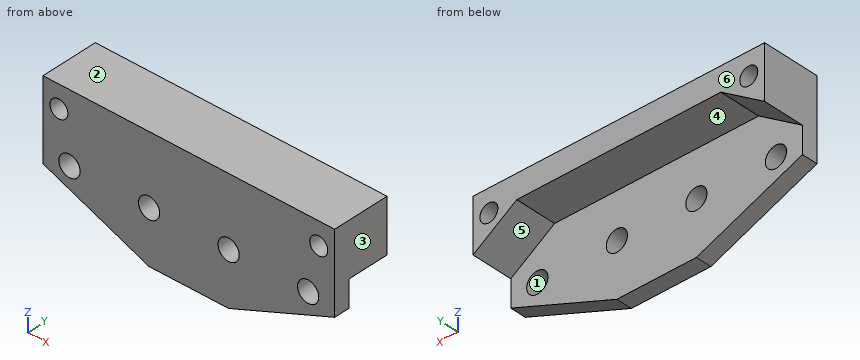
```python
from build123d import *

# Parameters (mm, degrees)
SKETCH2_R           = 2
BOSS_EXTRUDE1_DEPTH = 3
BOSS_EXTRUDE2_DEPTH = 7.8
SKETCH4_R           = 1.7
CUT_EXTRUDE1_DEPTH  = 61.585806919


with BuildPart() as part:
    # Sketch2 → Boss-Extrude1 (new body)
    with BuildSketch(Plane(origin=(0, 0, 0), x_dir=(1, 0, 0), z_dir=(0, 1, 0))):
        Polygon((0, 0), (0, 15), (20, 23), (35, 23), (55, 15), (55, 0), align=None)
        with Locations(Location((5, 13, 0), (0, 0, 270))):
            Circle(SKETCH2_R, mode=Mode.SUBTRACT)
        with Locations(Location((20, 13, 0), (0, 0, 270))):
            Circle(SKETCH2_R, mode=Mode.SUBTRACT)
        with Locations(Location((35, 13, 0), (0, 0, 270))):
            Circle(SKETCH2_R, mode=Mode.SUBTRACT)
        with Locations(Location((50, 13, 0), (0, 0, 270))):
            Circle(SKETCH2_R, mode=Mode.SUBTRACT)
    extrude(amount=BOSS_EXTRUDE1_DEPTH)

    # Sketch3 → Boss-Extrude2 (add)
    with BuildSketch(Plane(origin=(0, 3, 0), x_dir=(1, 0, 0), z_dir=(0, 1, 0))):
        Polygon((0, 10), (0, 0), (15, 0), (8.25, 4.5), align=None)
        Polygon((8.25, 4.5), (15, 0), (40, 0), (46.75, 4.5), align=None)
        Polygon((46.75, 4.5), (40, 0), (55, 0), (55, 10), align=None)
    extrude(amount=BOSS_EXTRUDE2_DEPTH)

    # Sketch4 → Cut-Extrude1 (cut, through all)
    with BuildSketch(Plane(origin=(0, 10.8, 0), x_dir=(1, 0, 0), z_dir=(0, 1, 0))):
        with Locations(Location((3, 4.25, 0), (0, 0, 270))):
            Circle(SKETCH4_R)
        with Locations(Location((52, 4.25, 0), (0, 0, 270))):
            Circle(SKETCH4_R)
    extrude(amount=-CUT_EXTRUDE1_DEPTH, mode=Mode.SUBTRACT)


solid = part.part
```
The model under review builds one solid part; all positions refer to its coordinate system, in mm. Face numbers are marked on the shaded views. A direction names the side the tool comes from. Coordinates: 2 decimals unless noted, no trailing zeros. Order: outer loops, then holes, each group sorted by start corner. A loop starts at its lowest first (then second) coordinate and runs counter-clockwise, first axis right, second up. Notation, with made-up numbers: (-10, 80) -> (20, 80) arc R23 ccw to (20, 100) -> close; hole circle Ø11 at (14.5, 68.5). An arc over 180 degrees is marked (long way). Answer in a Markdown table with one row per item. Add a question column.
Item 1: Machinability: for the marked faces 5 and 6, which of the approach directions +Z, -Z, +X, -X, +Y, -Y give a long, thin tool a straight path to every point of the face, cutting with its end or side? Answer none if there is none.
Item 2: We need section B-B on y = 8.75. Write out the cut boundary in (x, z).
Item 3: Mouldability with a two-part tool opening along Z and no side actions: class the marked faces 1, 2, 3 and 4 as +Z half, -Z half, draft (parallel to the pull), parting line (faces both ways), or undercut.
Item 4: We need section A-A on y = 1.25. Write out the cut boundary in (x, z), plus the area to 3 significant figures.
Item 5: Clearance check with flat-ended pins moving along their axes: pin 1 (4.5 mm diameter, centred on x = 5, z = -13, fed in from +Y); pin 2 (3 mm diameter, centred on x = 40, y = 8.5, fed in from -Z). State where each tip first meets the part, or that it passes through.
Item 6: We need section D-D on z = -11.5. Write out the cut boundary in (x, y).
Item 7: We need section C-C on x = 9.5. Write out the cut boundary in (y, z), plus the area to 3 significant figures.
Item 8: To check wall thickness, follow probe 1 along X at (y, z) = (2.3, -13); probe 2 along X at (y, z) = (5.25, -4.25); probe 3 along Y at (x, z) = (32, -21). State the ranges of each line that lie inside material, in increasing order.
Final values:
| question | item | result |
|---|---|---|
| 1 | face 5 | -Z, +Y |
| 1 | face 6 | +Z, -Z, +X, -X, +Y |
| 2 | outline | (0, -10) -> (8.25, -4.5) -> (46.75, -4.5) -> (55, -10) -> (55, 0) -> (0, 0) -> close; hole circle Ø3.4 at (3, -4.25); hole circle Ø3.4 at (52, -4.25) |
| 3 | face 1 | undercut |
| 3 | face 2 | +Z half |
| 3 | face 3 | draft |
| 3 | face 4 | -Z half |
| 4 | outline | (0, -15) -> (20, -23) -> (35, -23) -> (55, -15) -> (55, 0) -> (0, 0) -> close; hole circle Ø3.4 at (3, -4.25); hole circle Ø4 at (5, -13); hole circle Ø4 at (20, -13); hole circle Ø4 at (35, -13); hole circle Ø4 at (50, -13); hole circle Ø3.4 at (52, -4.25) |
| 4 | area | 1,040 mm2 |
| 5 | pin 1 | stops at y = 3 |
| 5 | pin 2 | stops at z = -4.5 |
| 6 | outline | (0, 0) -> (3.68, 0) -> (3.68, 3) -> (0, 3) -> close; (6.32, 0) -> (18.68, 0) -> (18.68, 3) -> (6.32, 3) -> close; (21.32, 0) -> (33.68, 0) -> (33.68, 3) -> (21.32, 3) -> close; (36.32, 0) -> (48.68, 0) -> (48.68, 3) -> (36.32, 3) -> close; (51.32, 0) -> (55, 0) -> (55, 3) -> (51.32, 3) -> close |
| 7 | outline | (0, -18.8) -> (3, -18.8) -> (3, -4.5) -> (10.8, -4.5) -> (10.8, 0) -> (0, 0) -> close |
| 7 | area | 91.5 mm2 |
| 8 | probe 1 | x = 0 to 3, 7 to 18, 22 to 33, 37 to 48, 52 to 55 |
| 8 | probe 2 | x = 0 to 1.3, 4.7 to 50.3, 53.7 to 55 |
| 8 | probe 3 | y = 0 to 3 |
